Check sheet for the modelled part. Datum: model origin and axes. Units: mm. Round coordinates to 2 decimals unless told otherwise and drop trailing zeros. Loops run counter-clockwise (first coordinate to the right, second up) from the corner with the lowest first, then second, coordinate; pieces in that order, holes last. Notation, with made-up numbers: M 70.5,-26.75 L 122.5,-26.75 A16 ccw 122.5,0.25 Z; hole C 21.5,66.5 d5. An arc over 180 degrees is marked long. Write item = value, one per line. Start each with the question number.
(1) Scan lines: L1, parallel to Z at x = 0.5, y = -1.3; L2, parallel to Z at x = -43, y = -0.9. Record each from-to range of solid material in increasing order. Write a range as from..to.
(2) Cross-section at C-C on z = -64.5. Record the boundary of the cut face in (x, y).
(3) Cross-section at B-B on z = 12.5. Record the boundary of the cut face in (x, y).
(4) Cross-section at A-A on y = -1.1. Record the boundary of the cut face in (x, z).
(5) Cross-section at D-D on x = 76.5. Record the boundary of the cut face in (y, z).
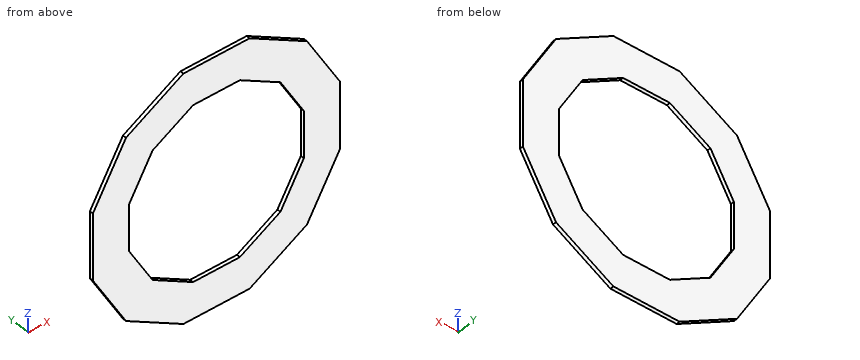
from build123d import *

# Parameters (mm, degrees)
BOSS_EXTRUDE1_DEPTH = 2.921
CUT_EXTRUDE1_DEPTH  = 139.818915977
BOSS_EXTRUDE2_DEPTH = 2.921


with BuildPart() as part:
    # Sketch1 → Boss-Extrude1 (new body)
    with BuildSketch(Plane(origin=(0, 0, 0), x_dir=(1, 0, 0), z_dir=(0, 1, 0))):
        Polygon((98.138063951, 26.296014982), (71.842048969, 71.842048969), (26.296014982, 98.138063951), (-26.296014982, 98.138063951), (-71.842048969, 71.842048969), (-98.138063951, 26.296014982), (-98.138063951, -26.296014982), (-71.842048969, -71.842048969), (-26.296014982, -98.138063951), (26.296014982, -98.138063951), (71.842048969, -71.842048969), (98.138063951, -26.296014982), align=None)
    extrude(amount=-BOSS_EXTRUDE1_DEPTH)

    # Sketch3 → Cut-Extrude1 (cut, through all)
    with BuildSketch(Plane(origin=(0, 0, 0), x_dir=(1, 0, 0), z_dir=(0, 1, 0))):
        Polygon((-71.395441524, 19.1303509), (-52.265090625, 52.265090625), (-19.1303509, 71.395441524), (19.1303509, 71.395441524), (52.265090625, 52.265090625), (71.395441524, 19.1303509), (71.395441524, -19.1303509), (52.265090625, -52.265090625), (19.1303509, -71.395441524), (-19.1303509, -71.395441524), (-52.265090625, -52.265090625), (-71.395441524, -19.1303509), align=None)
    extrude(amount=-CUT_EXTRUDE1_DEPTH, mode=Mode.SUBTRACT)

    # Sketch4 → Boss-Extrude2 (add)
    with BuildSketch(Plane(origin=(0, 0, 0), x_dir=(1, 0, 0), z_dir=(0, 1, 0))):
        Polygon((101.059063951, 27.078694574), (73.980369377, 73.980369377), (27.078694574, 101.059063951), (-27.078694574, 101.059063951), (-73.980369377, 73.980369377), (-101.059063951, 27.078694574), (-101.059063951, -27.078694574), (-73.980369377, -73.980369377), (-27.078694574, -101.059063951), (27.078694574, -101.059063951), (73.980369377, -73.980369377), (101.059063951, -27.078694574), align=None)
        Polygon((98.138063951, 26.296014982), (71.842048969, 71.842048969), (26.296014982, 98.138063951), (-26.296014982, 98.138063951), (-71.842048969, 71.842048969), (-98.138063951, 26.296014982), (-98.138063951, -26.296014982), (-71.842048969, -71.842048969), (-26.296014982, -98.138063951), (26.296014982, -98.138063951), (71.842048969, -71.842048969), (98.138063951, -26.296014982), align=None, mode=Mode.SUBTRACT)
    extrude(amount=-BOSS_EXTRUDE2_DEPTH)


solid = part.part
Result:
q1.L1 = -101.06..-71.4, 71.4..101.06
q1.L2 = -91.87..-57.61, 57.61..91.87
q2.outline = M -79.45,-2.92 L -31.07,-2.92 L -31.07,0 L -79.45,0 Z; M 31.07,-2.92 L 79.45,-2.92 L 79.45,0 L 31.07,0 Z
q3.outline = M -101.06,-2.92 L -71.4,-2.92 L -71.4,0 L -101.06,0 Z; M 71.4,-2.92 L 101.06,-2.92 L 101.06,0 L 71.4,0 Z
q4.outline = M -101.06,-27.08 L -73.98,-73.98 L -27.08,-101.06 L 27.08,-101.06 L 73.98,-73.98 L 101.06,-27.08 L 101.06,27.08 L 73.98,73.98 L 27.08,101.06 L -27.08,101.06 L -73.98,73.98 L -101.06,27.08 Z; hole M -71.4,-19.13 L -52.27,-52.27 L -19.13,-71.4 L 19.13,-71.4 L 52.27,-52.27 L 71.4,-19.13 L 71.4,19.13 L 52.27,52.27 L 19.13,71.4 L -19.13,71.4 L -52.27,52.27 L -71.4,19.13 Z
q5.outline = M -2.92,-69.62 L 0,-69.62 L 0,69.62 L -2.92,69.62 Z
